```python
from build123d import *

# Parameters (mm, degrees)
SKETCH1_W               = 25.4
SKETCH1_H               = 7.3
BOSS_EXTRUDE1_DEPTH     = 6
SKETCH3_W               = 4.4
SKETCH3_H               = 5.7
CUT_EXTRUDE1_DEPTH      = 21.24530815
CUT_EXTRUDE1_DEPTH_BACK = 21.24530815
BOSS_EXTRUDE3_START     = -3
BOSS_EXTRUDE3_DEPTH     = 3
BOSS_EXTRUDE4_START     = -3
BOSS_EXTRUDE4_DEPTH     = 3
FILLET1_R               = 1
CUT_EXTRUDE2_DEPTH      = 19.376955775
CUT_EXTRUDE3_DEPTH      = 19.376955775
SKETCH9_R               = 1.375
CUT_EXTRUDE4_DEPTH      = 8
CHAMFER1_SIZE           = 0.25


with BuildPart() as part:
    # Sketch1 → Boss-Extrude1 (new body)
    with BuildSketch(Plane.XY):
        Rectangle(SKETCH1_W, SKETCH1_H)
    extrude(amount=BOSS_EXTRUDE1_DEPTH)

    # Sketch2 → Revolve1 (revolve)
    with BuildSketch(Plane.XY.offset(3), mode=Mode.PRIVATE) as revolve1_sk:
        with BuildLine():
            Line((6.65, -6.15), (3, -6.15))
            Line((3, -6.15), (3, -3.65))
            Line((3, -3.65), (0, -3.65))
            Line((0, -3.65), (0, -11.85))
            Line((0, -11.85), (2.346446609, -11.85))
            ThreePointArc((2.346446609, -11.85), (2.729130042, -11.773879533), (3.053553391, -11.557106781))
            Line((3.053553391, -11.557106781), (7.180330086, -7.430330086))
            ThreePointArc((7.180330086, -7.430330086), (7.342909649, -6.612987426), (6.65, -6.15))
        make_face()
    revolve(revolve1_sk.sketch.rotate(Axis((0, 0, 3), (0, -1, 0)), 180), axis=Axis((0, 0, 3), (0, -1, 0)))

    # Sketch3 → Cut-Extrude1 (cut, two sides)
    with BuildSketch(Plane(origin=(0, 0, 0), x_dir=(0, 0, -1), z_dir=(1, 0, 0))) as cut_extrude1_sk:
        with Locations((-8.2, -9)):
            Rectangle(SKETCH3_W, SKETCH3_H)
        with Locations((2.2, -9)):
            Rectangle(SKETCH3_W, SKETCH3_H)
    extrude(amount=CUT_EXTRUDE1_DEPTH, mode=Mode.SUBTRACT)
    extrude(cut_extrude1_sk.sketch, amount=-CUT_EXTRUDE1_DEPTH_BACK, mode=Mode.SUBTRACT)

    # Sketch5 → Boss-Extrude3 (add)
    with BuildSketch(Plane(origin=(0, 0, 0), x_dir=(-1, 0, 0), z_dir=(0, 0, -1)).offset(BOSS_EXTRUDE3_START)):
        with BuildLine():
            Line((-7.180330086, -7.430330086), (-3.053553391, -11.557106781))
            ThreePointArc((-3.053553391, -11.557106781), (-2.729130042, -11.773879533), (-2.346446609, -11.85))
            Line((-2.346446609, -11.85), (0, -11.85))
            Line((0, -11.85), (0, -6.15))
            Line((0, -6.15), (-6.65, -6.15))
            ThreePointArc((-6.65, -6.15), (-7.342909649, -6.612987426), (-7.180330086, -7.430330086))
        make_face()
    extrude(amount=BOSS_EXTRUDE3_DEPTH)

    # Sketch6 → Boss-Extrude4 (add)
    with BuildSketch(Plane.XY.offset(6).offset(BOSS_EXTRUDE4_START)):
        with BuildLine():
            Line((0, -11.85), (0, -11.606880417))
            add(Edge.make_bspline(
                [(-0.569375368, -11.557106781), (-0.477136244, -11.574305984), (-0.383216001, -11.587587431), (-0.288131205, -11.597299525), (-0.192322641, -11.603685849), (-0.096171282, -11.606880411), (0, -11.606880417)],
                knots=[0, 0, 0, 0, 0, 0, 0, 0.500004034, 0.500004034, 0.500004034, 0.500004034, 0.500004034, 0.500004034, 0.500004034], degree=6))
            add(Edge.make_bspline(
                [(-0.569375368, -11.557106781), (-2.345972894, -11.225836703), (-6.523583382, -7.430330086)],
                knots=[0.188670459, 0.188670459, 0.188670459, 1.519069158, 1.519069158, 1.519069158], degree=2, weights=[1, 1.229524605, 1]))
            add(Edge.make_bspline(
                [(-6.523583382, -7.430330086), (-6.548217839, -7.407948812), (-6.57163623, -7.384387754), (-6.593752622, -7.359710949), (-6.614485917, -7.333990738), (-6.633761234, -7.307307749), (-6.688090057, -7.222962512), (-6.718198081, -7.1624526), (-6.741231365, -7.099013892), (-6.756763407, -7.033555882), (-6.764556488, -6.967070385), (-6.764657168, -6.849785487), (-6.760183262, -6.798976266), (-6.751191088, -6.748616972), (-6.737758143, -6.699153447), (-6.720033498, -6.651010063), (-6.68841653, -6.583676772), (-6.677775298, -6.563121343), (-6.666326858, -6.542947595), (-6.654092776, -6.523189068), (-6.641096757, -6.503877463), (-6.605240936, -6.454697957), (-6.581206245, -6.425590465), (-6.555368287, -6.397845087), (-6.527846234, -6.371572034), (-6.498768133, -6.346867107), (-6.393778747, -6.267504617), (-6.310809109, -6.22103841), (-6.221317835, -6.185601518), (-6.127427397, -6.161840052), (-6.031244011, -6.15), (-5.934854674, -6.15)],
                knots=[0, 0, 0, 0, 0, 0, 0, 0.107806274, 0.107806274, 0.107806274, 0.107806274, 0.107806274, 0.32997016, 0.32997016, 0.32997016, 0.32997016, 0.32997016, 0.499739877, 0.499739877, 0.499739877, 0.499739877, 0.499739877, 0.576163763, 0.576163763, 0.576163763, 0.576163763, 0.576163763, 0.699289859, 0.699289859, 0.699289859, 0.699289859, 0.699289859, 1, 1, 1, 1, 1, 1, 1], degree=6))
            Line((-5.934854674, -6.15), (-6.65, -6.15))
            ThreePointArc((-6.65, -6.15), (-7.342909649, -6.612987426), (-7.180330086, -7.430330086))
            Line((-7.180330086, -7.430330086), (-3.053553391, -11.557106781))
            ThreePointArc((-3.053553391, -11.557106781), (-2.729130042, -11.773879533), (-2.346446609, -11.85))
            Line((-2.346446609, -11.85), (0, -11.85))
        make_face()
    extrude(amount=BOSS_EXTRUDE4_DEPTH)

    # Fillet1
    fillet1_edges = [part.edges().sort_by_distance(p)[0] for p in [
        (12.7, -3.65, 3),
        (-12.7, -3.65, 3),
        (-12.7, 3.65, 3),
        (12.7, 3.65, 3),
    ]]
    fillet(fillet1_edges, radius=FILLET1_R)

    # Sketch7 → Cut-Extrude2 (cut, through all)
    with BuildSketch(Plane.ZY):
        with BuildLine():
            Line((0, -11.606880417), (0, -11.85))
            Line((0, -11.85), (0.653553391, -11.85))
            ThreePointArc((0.653553391, -11.85), (0.304899133, -11.787251412), (0, -11.606880417))
        make_face()
    extrude(amount=-CUT_EXTRUDE2_DEPTH, mode=Mode.SUBTRACT)

    # Sketch8 → Cut-Extrude3 (cut, through all)
    with BuildSketch(Plane(origin=(0, 0, 0), x_dir=(0, 0, -1), z_dir=(1, 0, 0))):
        with BuildLine():
            Line((-6, -11.606880417), (-6, -11.85))
            Line((-6, -11.85), (-5.346446609, -11.85))
            ThreePointArc((-5.346446609, -11.85), (-5.695100867, -11.787251412), (-6, -11.606880417))
        make_face()
    extrude(amount=-CUT_EXTRUDE3_DEPTH, mode=Mode.SUBTRACT)

    # Sketch9 → Cut-Extrude4 (cut)
    with BuildSketch(Plane(origin=(0, 3.65, 0), x_dir=(1, 0, 0), z_dir=(0, 1, 0))):
        with Locations(Location((0, -3, 0), (0, 0, 270))):
            Circle(SKETCH9_R)
    extrude(amount=-CUT_EXTRUDE4_DEPTH, mode=Mode.SUBTRACT)

    # Chamfer1
    chamfer1_edges = [part.edges().sort_by_distance(p)[0] for p in [
        (0, 3.65, 1.625),
    ]]
    chamfer(chamfer1_edges, length=CHAMFER1_SIZE)


solid = part.part
```
Design review of the part built by this model. Coordinates are the model's own, in mm. Round coordinates to 2 decimals unless told otherwise and drop trailing zeros. Write each loop counter-clockwise with the first axis right and the second up, starting at its lowest first coordinate (ties: lowest second). Pieces come first, ordered by that corner, then holes. Notation, with made-up numbers: (48.25, 72) -> (89.25, 72) arc R29 cw to (89.25, 101) -> close; hole circle Ø5 at (51.25, 10). An arc over 180 degrees is marked (long way). Write item = value, one per line. Start each with the question number.
1) Wall thickness on probe 1 along X at (y, z) = (-0.5, 3) (3 decimals); probe 2 along Y at (x, z) = (7.5, 4); probe 3 along Z at (x, y) = (2.5, -10.75): over which ranges is each line inside the solid? List them lowest first. Write a range as from..to.
2) Clearance check with flat-ended pins moving along their axes: pin 1 (1.8 mm diameter, centred on x = -4.5, z = 4, fed in from -Y); pin 2 (1.4 mm diameter, centred on x = -0.5, z = 3, fed in from +Y). State where each tip first meets the part, or that it passes through.
3) Take a section at D-D, the plane y = -10.25. State the section outline as (x, z) points, plus the area to 3 significant figures.
4) Take a section at C-C, the plane y = -5.25. State the section outline as (x, z) points.
5) Take a section at B-B, the plane x = -7.75. State the section outline as (y, z) points.
6) Mouldability with a two-part tool opening along Y and no side actions: class faces 1 (the face through (-1.384, -4.882, 5.662)), 2 (the face through (0, -8, 0)), 3 (the face through (4.362, -9.923, 4.715)) as +Y half, -Y half, draft (parallel to the pull), parting line (faces both ways), or undercut.
7) Take a section at A-A, the plane y = -2.25. State the section outline as (x, z) points (3 decimals).
Results list:
q1.probe_1 = -12.7..-1.375, 1.375..12.7
q1.probe_2 = -3.65..3.65
q1.probe_3 = 0..5.94
q2.pin_1 = -11.01
q2.pin_2 = -4.35
q3.outline = (-4.36, 3) arc R4.36 ccw to (-3.16, 0) -> (4.36, 0) -> (4.36, 3) arc R4.36 ccw to (3.16, 6) -> (-4.36, 6) -> close
q3.area = 50.1 mm²
q4.outline = circle Ø6 at (0, 3)
q5.outline = (-3.65, 0) -> (3.65, 0) -> (3.65, 6) -> (-3.65, 6) -> close
q6.face_1 = undercut
q6.face_2 = draft
q6.face_3 = -Y half
q7.outline = (-12.7, 0) -> (12.7, 0) -> (12.7, 6) -> (-12.7, 6) -> close; hole circle Ø2.75 at (0, 3)
